For this review, take the finished solid that the model builds, in its own axes (mm). A direction names the side the tool comes from. Coordinates: 2 decimals unless noted, no trailing zeros. Write each loop counter-clockwise with the first axis right and the second up, starting at its lowest first coordinate (ties: lowest second). Pieces come first, ordered by that corner, then holes.
```python
from build123d import *

# Parameters (mm, degrees)
SKETCH_W     = 123.756
SKETCH_H     = 79
PAD_DEPTH    = 3
SKETCH001_W  = 2
SKETCH001_H  = 11
PAD001_DEPTH = 5
SKETCH002_W  = 11
SKETCH002_H  = 2.5
PAD002_DEPTH = 4
SKETCH003_W  = 2
SKETCH003_H  = 11
PAD003_DEPTH = 2
FILLET_R     = 1


with BuildPart() as part:
    # Sketch → Pad (new body)
    with BuildSketch(Plane.XY):
        Rectangle(SKETCH_W, SKETCH_H)
    extrude(amount=PAD_DEPTH)

    # Sketch001 (on Face5 of Pad) → Pad001 (join)
    with BuildSketch(Plane(origin=(0, 0, 0), x_dir=(1, 0, 0), z_dir=(0, 0, -1))):
        Rectangle(SKETCH001_W, SKETCH001_H)
    extrude(amount=PAD001_DEPTH)

    # Sketch002 (on Face7 of Pad001) → Pad002 (join)
    with BuildSketch(Plane(origin=(-1, 0, 0), x_dir=(0, -1, 0), z_dir=(-1, 0, 0))):
        with Locations((0, -3.75)):
            Rectangle(SKETCH002_W, SKETCH002_H)
    extrude(amount=PAD002_DEPTH)

    # Sketch003 (on Face16 of Pad002) → Pad003 (join)
    with BuildSketch(Plane(origin=(0, 0, -2.5), x_dir=(1, 0, 0), z_dir=(0, 0, -1))):
        with Locations((-4, 0)):
            Rectangle(SKETCH003_W, SKETCH003_H)
    extrude(amount=-PAD003_DEPTH)

    # Fillet
    fillet_edges = [part.edges().sort_by_distance(p)[0] for p in [
        (1, -5.5, -2.5),
        (1, 5.5, -2.5),
        (1, 0, 0),
        (1, 0, -5),
        (0, -5.5, -5),
        (0, 5.5, -5),
        (-1, 0, -5),
        (-3, -5.5, -5),
        (-3, 5.5, -5),
        (-5, 0, -5),
        (-5, 0, -2.5),
        (-5, -5.5, -3.75),
        (-5, 5.5, -3.75),
        (-5, 5.5, -1.5),
        (-5, -5.5, -1.5),
        (-5, 0, -0.5),
    ]]
    fillet(fillet_edges, radius=FILLET_R)


solid = part.part
```
Q1. Draft analysis for pull direction X (two halves, no side actions). For faces 5 (the flat face through (-2, -5.5, -3)), 6 (the flat face through (61.878, -1, 1)), 7 (the flat face through (-1, 0, -1)), 8 (the flat face through (-61.878, -1, 1)), state which applies: +X half, -X half, draft (parallel to the pull), parting line (faces both ways), or undercut.
Ans:
face 5: draft
face 6: +X half
face 7: undercut
face 8: -X half
Q2. Clearance check with flat-ended pins moving along their axes: pin 1 Ø3 at (y, z) = (-1, -3.5) entering from -X; pin 2 Ø2 at (x, y) = (35.5, -30) entering from -Z; pin 3 Ø2 at (y, z) = (0, -1.5) entering from +X. State where each tip first meets the part, or that it passes through.
Ans:
pin 1: stops at x = -5
pin 2: stops at z = 0
pin 3: stops at x = 1.13
Q3. Add section A-A (y = 15). State the section outline as (x, z) points, then the cut area to 3 significant figures.
Ans:
outline: (-61.88, 0) - (61.88, 0) - (61.88, 3) - (-61.88, 3) - close
area: 371 mm2
Q4. Tool access review of faces 1 (the flat face through (1, 0, -2)), 2 (the flat face through (-2, 5.5, -3)), 3 (the flat face through (-5, 0, -3)), 4 (the flat face through (-1, 39.5, 1)): name each direction out of +Z, -Z, +X, -X, +Y, -Y from which nothing blocks a thin tool from reaching the whole face with its end or side.
Ans:
face 1: -Z, +X, +Y, -Y
face 2: -Z, +X, -X, +Y
face 3: -Z, -X, +Y, -Y
face 4: +Z, -Z, +X, -X, +Y
Q5. Add section B-B (x = -32). State the section outline as (y, z) points.
Ans:
outline: (-39.5, 0) - (39.5, 0) - (39.5, 3) - (-39.5, 3) - close
Q6. For probe 1 along Z at (x, y) = (40.5, 15); probe 2 along Y at (x, z) = (-4, -3); probe 3 along X at (y, z) = (-1, -0.75), list the stretches that pass through material, from the lowest coordinate up.
Ans:
probe 1: z = 0 to 3
probe 2: y = -5.5 to 5.5
probe 3: x = -4.66 to -3, -1 to 1.03
